Work out the finished part from the listing and answer in its coordinate system (mm). A direction names the side the tool comes from. Give positions to 0.01 mm unless a question says otherwise; leave off trailing zeros. Loops run counter-clockwise (first coordinate to the right, second up) from the corner with the lowest first, then second, coordinate; pieces in that order, holes last. Notation, with made-up numbers: (32.5, 10) - (57.5, 10) arc R14 cw to (57.5, 15) - close; hole circle Ø1 at (-3, -23). An arc over 180 degrees is marked (long way). Use CSV: the item, a comma, the result in double quotes.
from build123d import *

# Parameters (mm, degrees)
SKETCH_1_R      = 4
EXTRUDE_1_DEPTH = 117.5
SKETCH_2_W      = 0.5
SKETCH_2_H      = 1


with BuildPart() as part:
    # Sketch 1 → Extrude 1 (new body)
    with BuildSketch(Plane.XY):
        with Locations(Location((0, 0, 0), (0, 0, 180))):
            Circle(SKETCH_1_R)
    extrude(amount=EXTRUDE_1_DEPTH)

    # Sketch 2 → Cut-Revolve 1 (revolve, cut)
    with BuildSketch(Plane(origin=(0, 0, 0), x_dir=(1, 0, 0), z_dir=(0, 1, 0)), mode=Mode.PRIVATE) as cut_revolve_1_sk:
        with Locations((3.75, -2.5)):
            Rectangle(SKETCH_2_W, SKETCH_2_H)
        with Locations((3.75, -115)):
            Rectangle(SKETCH_2_W, SKETCH_2_H)
    revolve(cut_revolve_1_sk.sketch.rotate(Axis((0, 0, 117.5), (0, 0, -1)), 180), axis=Axis((0, 0, 117.5), (0, 0, -1)), mode=Mode.SUBTRACT)


solid = part.part
Item 1: A cutting plane is placed at B-B on z = 29.5. Determine the outline of the cut face in (x, y), and give its area (3 significant figures).
Determined:
outline,"circle Ø8 at (0, 0)"
area,"50.3 mm²"
Item 2: Find the intervals of material crossed by line 1 (Z direction, x = -3.5, y = 1.5); line 2 (Y direction, x = -0.5, z = 50); line 3 (X direction, y = -2, z = 57), in increasing order.
Determined:
line 1,"z = 0 to 2, 3 to 114.5, 115.5 to 117.5"
line 2,"y = -3.97 to 3.97"
line 3,"x = -3.46 to 3.46"
Item 3: For faces 1 (the cylindrical face through (-3.233, -1.341, 114.993)), 2 (the cylindrical face through (0.867, 3.905, 57.97)), determine the directions among +Z, -Z, +X, -X, +Y, -Y from which every point of the face is accessible in a straight line to the end or side of a thin tool.
Determined:
face 1,"none"
face 2,"+Z, -Z"
Item 4: The mould has two halves that part along Z. Classify faces 3 (the cylindrical face through (-3.233, -1.341, 2.493)), 4 (the cylindrical face through (0.867, 3.905, 116.486)), 5 (the flat face through (0, 0, 0)): pulls with the +Z half, pulls with the -Z half, needs draft (parallel to the pull), parting line crosses it, or undercut.
Determined:
face 3,"undercut"
face 4,"needs draft"
face 5,"pulls with the -Z half"
Item 5: Given P1, Ø1, axis at x = -2, z = 45.5, coming from the +Y side, flat-ended and moving along its own axis, determine where the tip first touches the part or whether it passes through.
Determined:
P1,"stops at y = 3.71"
Item 6: A cutting plane is placed at A-A on y = 1. Determine the outline of the cut face in (x, z), and give its area (3 significant figures).
Determined:
outline,"(-3.87, 0) - (3.87, 0) - (3.87, 2) - (3.35, 2) - (3.35, 3) - (3.87, 3) - (3.87, 114.5) - (3.35, 114.5) - (3.35, 115.5) - (3.87, 115.5) - (3.87, 117.5) - (-3.87, 117.5) - (-3.87, 115.5) - (-3.35, 115.5) - (-3.35, 114.5) - (-3.87, 114.5) - (-3.87, 3) - (-3.35, 3) - (-3.35, 2) - (-3.87, 2) - close"
area,"908 mm²"
